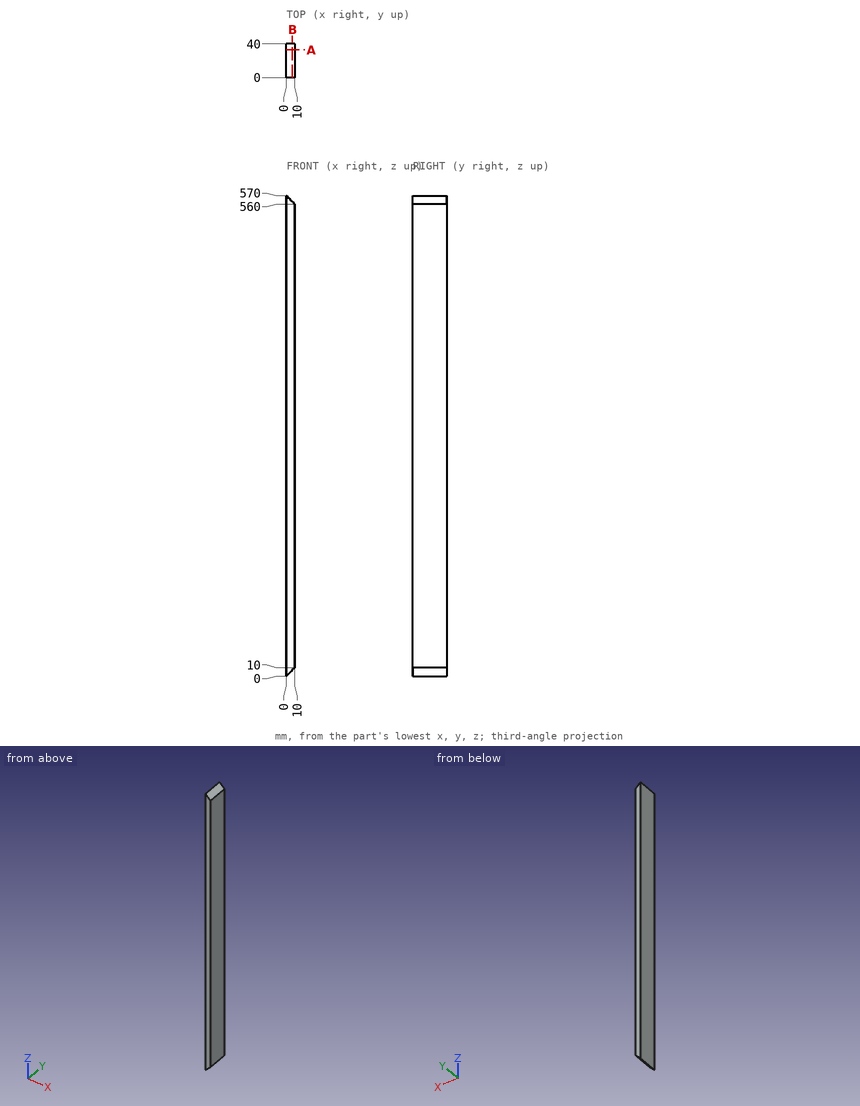
Design review of the part shown in the three views and the two pictorial views. Dimensions are in mm from the part's minimum x, y and z. Round coordinates to 2 decimals unless told otherwise and drop trailing zeros. Loops run counter-clockwise (first coordinate to the right, second up) from the corner with the lowest first, then second, coordinate; pieces in that order, holes last. Notation, with made-up numbers: (-13, 3) - (10, 3) arc R26 cw to (10, 21) - close; hole circle Ø11 at (13, 17). An arc over 180 degrees is marked (long way). Answer as CSV lines item,"result".
(1) Insertion check: P1, Ø3, axis at x = 4, y = 14.5, coming from the -Z side; P2, Ø2, axis at x = 4.5, y = 17, coming from the +Z side. Each pin has a flat end and moves straight along its axis. Give the tip position at first contact, or say it passes through.
Checked values:
P1,"stops at z = 2.5"
P2,"stops at z = 566.5"
(2) Wall thickness on line 1 (Z direction, x = 0.5, y = 19); line 2 (Z direction, x = 8.25, y = 4): over which ranges is each line inside the solid? List them lowest first.
Checked values:
line 1,"z = 0.5 to 569.5"
line 2,"z = 8.25 to 561.75"
(3) Consider section A-A on y = 33. Give the boundary of the cut face in (x, z).
Checked values:
outline,"(0, 0) - (10, 10) - (10, 560) - (0, 570) - close"
(4) Consider section B-B on x = 7. Give the boundary of the cut face in (y, z).
Checked values:
outline,"(0, 7) - (40, 7) - (40, 563) - (0, 563) - close"
